```python
from build123d import *

# Parameters (mm, degrees)
SKETCH_R        = 15
PAD_DEPTH       = 6
FILLET_R        = 1
FILLET001_R     = 1
SKETCH001_R     = 12.5
POCKET_DEPTH    = 3
PAD001_DEPTH    = 25
SKETCH003_R     = 1.55
POCKET001_DEPTH = 20
SKETCH004_R     = 1
POCKET002_DEPTH = 6


with BuildPart() as part:
    # Sketch → Pad (new body)
    with BuildSketch(Plane.XY):
        Circle(SKETCH_R)
    extrude(amount=PAD_DEPTH)

    # Fillet
    fillet_edges = [part.edges().sort_by_distance(p)[0] for p in [
        (-15, 0, 0),
    ]]
    fillet(fillet_edges, radius=FILLET_R)

    # Fillet001
    fillet001_edges = [part.edges().sort_by_distance(p)[0] for p in [
        (-15, 0, 6),
    ]]
    fillet(fillet001_edges, radius=FILLET001_R)

    # Sketch001 (on Face4 of Fillet001) → Pocket (cut)
    with BuildSketch(Plane.XY.offset(6)):
        Circle(SKETCH001_R)
    extrude(amount=-POCKET_DEPTH, mode=Mode.SUBTRACT)

    # Sketch002 (on Face7 of Pocket) → Pad001 (join)
    with BuildSketch(Plane.XY.offset(3)):
        with BuildLine():
            Line((-3, 12.134661), (-3, -12.134661))
            ThreePointArc((-3, -12.134661), (0, -12.5), (3, -12.134661))
            Line((3, 12.134661), (3, -12.134661))
            ThreePointArc((3, 12.134661), (0, 12.5), (-3, 12.134661))
        make_face()
    extrude(amount=PAD001_DEPTH)

    # Sketch003 (on Face11 of Pad001) → Pocket001 (cut)
    with BuildSketch(Plane.YZ.offset(3)):
        with Locations((0, 23)):
            Circle(SKETCH003_R)
        with Locations((0, 15)):
            Circle(SKETCH003_R)
    extrude(amount=-POCKET001_DEPTH, mode=Mode.SUBTRACT)

    # Sketch004 (on Face3 of Pad) → Pocket002 (cut)
    with BuildSketch(Plane.XY.offset(6)):
        with Locations((-5.656854, 5.656854)):
            Circle(SKETCH004_R)
        with Locations((5.656854, 5.656854)):
            Circle(SKETCH004_R)
        with Locations((-5.656854, -5.656854)):
            Circle(SKETCH004_R)
        with Locations((5.656854, -5.656854)):
            Circle(SKETCH004_R)
    extrude(amount=-POCKET002_DEPTH, mode=Mode.SUBTRACT)


solid = part.part
```
Read the model definition and answer for the solid it produces. Units are mm, in the model's axes. A direction names the side the tool comes from. Coordinates: 2 decimals unless noted, no trailing zeros. Loops run counter-clockwise (first coordinate to the right, second up) from the corner with the lowest first, then second, coordinate; pieces in that order, holes last.
(1) A tool of negligible diameter and unlimited length cuts with its end or side. For faces 1 (the face through (-7, 0, 3)), 2 (the face through (0.042, -0.202, 16.537)), 3 (the face through (0, 12.5, 16.8)), from which of +Z, -Z, +X, -X, +Y, -Y can it reach the whole face along a straight path? Write none if from no direction.
Solution:
face 1: +Z
face 2: +X, -X
face 3: +Z, +Y
(2) The part is cut by section A-A (z = 15). Determine the outline of the cut face in (x, y), and give its area (3 significant figures).
Solution:
outline: (-3, -12.13) arc R12.5 ccw to (3, -12.13) - (3, -1.55) - (-3, -1.55) - close; (-3, 1.55) - (3, 1.55) - (3, 12.13) arc R12.5 ccw to (-3, 12.13) - close
area: 130 mm2
(3) The part is cut by section C-C (x = 0). Determine the outline of the cut face in (y, z).
Solution:
outline: (-15, 1) arc R1 ccw to (-14, 0) - (14, 0) arc R1 ccw to (15, 1) - (15, 5) arc R1 ccw to (14, 6) - (12.5, 6) - (12.5, 28) - (-12.5, 28) - (-12.5, 6) - (-14, 6) arc R1 ccw to (-15, 5) - close; hole circle Ø3.1 at (0, 15); hole circle Ø3.1 at (0, 23)
(4) The part is cut by section D-D (z = 4.5). Determine the outline of the cut face in (x, y), and give its area (3 significant figures).
Solution:
outline: circle Ø30 at (0, 0); hole (-3, -12.13) - (-3, 12.13) arc R12.5 ccw to start; hole (3, -12.13) arc R12.5 ccw to (3, 12.13) - close
area: 365 mm2
(5) The part is cut by section B-B (y = 0). Determine the outline of the cut face in (x, z), and give its area (3 significant figures).
Solution:
outline: (-15, 1) arc R1 ccw to (-14, 0) - (14, 0) arc R1 ccw to (15, 1) - (15, 5) arc R1 ccw to (14, 6) - (12.5, 6) - (12.5, 3) - (3, 3) - (3, 13.45) - (-3, 13.45) - (-3, 3) - (-12.5, 3) - (-12.5, 6) - (-14, 6) arc R1 ccw to (-15, 5) - close; (-3, 16.55) - (3, 16.55) - (3, 21.45) - (-3, 21.45) - close; (-3, 24.55) - (3, 24.55) - (3, 28) - (-3, 28) - close
area: 217 mm2
(6) Flat-ended cylindrical pins translate along their axes: pin 1 Ø2.5 at (y, z) = (0, 15) entering from -X; pin 2 Ø2.5 at (x, y) = (5.66, -5.66) entering from +Z; pin 3 Ø7.5 at (x, y) = (-9.5, 0.5) entering from +Z; pin 4 Ø4 at (y, z) = (-8, 6.5) entering from +X. Find the tip coordinate at first contact, or state that the pin passes through.
Solution:
pin 1: passes through
pin 2: stops at z = 3
pin 3: stops at z = 6
pin 4: stops at x = 13.52
(7) Consider line 1 along Z through (x, y) = (0.85, 0); line 2 along X through (y, z) = (9.5, 23.5); line 3 along Z through (x, y) = (-11.25, 1.25). Determine where each line is inside the solid, lowest interval first.
Solution:
line 1: z = 0 to 13.45, 16.55 to 21.45, 24.55 to 28
line 2: x = -3 to 3
line 3: z = 0 to 3
(8) The mould has two halves that part along Y. Classify faces 4 (the face through (0, 0, 28)), 5 (the face through (12.5, -0.2, 4.5)), 6 (the face through (0, -12.5, 16.8)): released by +Y, released by -Y, zero draft, split by the parting line, or undercut.
Solution:
face 4: zero draft
face 5: undercut
face 6: released by -Y
